Autodesk Inventor part; units mm, degrees
ref_plane "YZ Plane" through (0, 0, 0) normal (1, 0, 0) x (0, 1, 0)
ref_plane "XZ Plane" through (0, 0, 0) normal (0, 1, 0) x (-1, 0, 0)
ref_plane "XY Plane" through (0, 0, 0) normal (0, 0, 1) x (1, 0, 0)
sketch "Boceto1" plane through (0, 0, 0) normal (0, 0, 1) x (1, 0, 0)
  circle A0 centre (0, 0) radius 5
  dimension "d0" = 10
extrude "Cuerpo manija" add sketch "Boceto1" along normal mid plane 95
sketch "Boceto2" plane through (0, 0, 47.5) normal (0, 0, 1) x (1, 0, 0)
  circle A0 centre (0, 0) radius 5
hole "M5X0.7 15" at (0, 0, 47.5) direction (0, 0, -1) diameter 4.134 depth 15 tip angle 118
sketch "Boceto3" plane through (0, 0, -47.5) normal (0, 0, -1) x (-1, 0, 0)
  point P0 (0, 0)
  point P1 (0, 0)
hole "M%X0.7 P15" at (0, 0, -47.5) direction (0, 0, 1) diameter 4.134 depth 15 tip angle 118
properties part number "eje"
Input: part model. Units: mm. Frame: model coordinates. A direction names the side the tool comes from. Round coordinates to 2 decimals unless told otherwise and drop trailing zeros. Loops run counter-clockwise (first coordinate to the right, second up) from the corner with the lowest first, then second, coordinate; pieces in that order, holes last. Notation, with made-up numbers: M 78.5,8.25 L 128.5,8.25 A7 cw 128.5,12.25 Z; hole C 21.25,85 d2. An arc over 180 degrees is marked long. Answer in a Markdown table with one row per item. Add a question column.
1. Mould query, pull axis X, two halves, no side actions, for faces 1 (the face through (2, -1, -47.5)), 2 (the face through (0.108, -0.342, 31.474)), 3 (the face through (1.26, 1.64, 39.89)), 4 (the face through (-1.08, 4.88, -0.66)). Classes: released by +X, released by -X, zero draft, split by the parting line, or undercut.
2. Section A-A (z = 35.5). Output: boundary loops of the cut face in (x, y).
3. Ray query, probe 1 along Y at (x, z) = (0, -39.5); probe 2 along X at (y, z) = (-0.25, -36); probe 3 along Y at (x, z) = (-0.5, -37). Return the intervals inside material, ascending.
4. Section C-C (y = -3). Output: boundary loops of the cut face in (x, z), and give its area (3 significant figures).
5. Section D-D (z = -27.5). Output: boundary loops of the cut face in (x, y).
6. Contact query for flat-ended pins moving along their axis: pin 1 (3.5 mm diameter, centred on x = 0, y = 0, fed in from +Z); pin 2 (1 mm diameter, centred on x = 0.5, z = 30, fed in from +Y); pin 3 (2 mm diameter, centred on x = -2.5, z = -17, fed in from +Y); pin 4 (2 mm diameter, centred on x = -4, z = 9.5, fed in from -Y). Output: stop coordinate, or through.
7. Set-up query: faces 5 (the face through (1.26, -1.64, -39.89)), 6 (the face through (2, -1, 47.5)). Return all of +Z, -Z, +X, -X, +Y, -Y with unobstructed straight access to the full face (end or side cutting, diameter ignored); none if empty.
8. Section B-B (x = 4). Output: boundary loops of the cut face in (y, z), and give its area (3 significant figures).
Values follow:
| question | item | result |
|---|---|---|
| 1 | face 1 | zero draft |
| 1 | face 2 | undercut |
| 1 | face 3 | undercut |
| 1 | face 4 | split by the parting line |
| 2 | outline | C 0,0 d10; hole C 0,0 d4.13 |
| 3 | probe 1 | -5 to -2.07, 2.07 to 5 |
| 3 | probe 2 | -4.99 to -2.05, 2.05 to 4.99 |
| 3 | probe 3 | -4.97 to -2.01, 2.01 to 4.97 |
| 4 | outline | M -4,-47.5 L 4,-47.5 L 4,47.5 L -4,47.5 Z |
| 4 | area | 760 mm^2 |
| 5 | outline | C 0,0 d10 |
| 6 | pin 1 | z = 32.31 |
| 6 | pin 2 | y = 5 |
| 6 | pin 3 | y = 4.77 |
| 6 | pin 4 | y = -4 |
| 7 | face 5 | -Z |
| 7 | face 6 | +Z, +X, -X, +Y, -Y |
| 8 | outline | M -3,-47.5 L 3,-47.5 L 3,47.5 L -3,47.5 Z |
| 8 | area | 570 mm^2 |
